from build123d import *

# Parameters (mm, degrees)
SKETCH1_R               = 15
BOSS_EXTRUDE1_DEPTH     = 35
SHELL1_T                = -2
ADVANCEDHOLE1_OUTLINE_R = 3
ADVANCEDHOLE1_DEPTH     = 2


# Read off the part's stored shape, not the designer's step: AdvancedHole1
with BuildPart() as part:
    # Sketch1 → Boss-Extrude1 (new body)
    with BuildSketch(Plane(origin=(0, 0, 0), x_dir=(1, 0, 0), z_dir=(0, 1, 0))):
        with Locations(Location((-13.930579922, 15.357614938, 0), (0, 0, 270))):
            Circle(SKETCH1_R)
    extrude(amount=BOSS_EXTRUDE1_DEPTH)

    # Shell1
    shell1_openings = [part.faces().sort_by_distance(p)[0] for p in [
        (-13.930579922, 35, -15.357614938),
    ]]
    offset(amount=SHELL1_T, openings=shell1_openings, kind=Kind.INTERSECTION)

    # AdvancedHole1 outline → AdvancedHole1 (cut)
    with BuildSketch(Plane(origin=(0, 0, 0), x_dir=(1, 0, 0), z_dir=(0, 1, 0))):
        with Locations((-13.850292644, 15.457974035)):
            Circle(ADVANCEDHOLE1_OUTLINE_R)
    extrude(amount=ADVANCEDHOLE1_DEPTH, mode=Mode.SUBTRACT)


solid = part.part
The model under review builds one solid part; all positions refer to its coordinate system, in mm. A direction names the side the tool comes from. Give positions to 0.01 mm unless a question says otherwise; leave off trailing zeros. Write each loop counter-clockwise with the first axis right and the second up, starting at its lowest first coordinate (ties: lowest second). Pieces come first, ordered by that corner, then holes. Notation, with made-up numbers: M 64.5,3 L 80.5,3 A30 cw 80.5,38 Z; hole C 77,-19.5 d9. An arc over 180 degrees is marked long. One line per question, with ' | ' between items. Start each with the question number.
Item 1: We need section B-B on x = -12.75. Write out the cut boundary in (y, z).
Item 2: We need section C-C on x = -19.75. Write out the cut boundary in (y, z), plus the area to 3 significant figures.
Item 3: Wall thickness on line 1 (X direction, y = 4, z = -15.25); line 2 (Y direction, x = -13.5, z = -6.5); line 3 (X direction, y = 17, z = -6.25): over which ranges is each line inside the solid? List them lowest first. Write a range as from..to.
Item 4: We need section D-D on z = -6.75. Write out the cut boundary in (x, y).
Item 5: For faces 5 (the flat face through (-17, 2, -13)), 6 (the flat face through (-7, 35, -27)), list the 3-axis set-ups (+Z, -Z, +X, -X, +Y, -Y) from which the entire face can be reached by the end or side of a thin tool; tool diameter is ignored.
Item 6: Draft analysis for pull direction X (two halves, no side actions). For faces 1 (the cylindrical face through (-3.79, 17.26, -26.41)), 2 (the cylindrical face through (-16.23, 0.99, -13.63)), 3 (the cylindrical face through (-21.841, 18.269, -25.674)), 4 (the flat face through (-14, 0, -12)), state which applies: released by +X, released by -X, zero draft, split by the parting line, or undercut.
Item 7: We need section A-A on z = -14.5. Write out the cut boundary in (x, y), plus the area to 3 significant figures.
Item 8: For pin 1 (6 mm diameter, centred on x = -20.5, y = 19, fed in from +Z); pin 2 (6 mm diameter, centred on y = 19, z = -4, fed in from +X); pin 3 (3 mm diameter, centred on x = -9.5, y = 5, fed in from -Z), all flat-tipped, find the tip position at first contact; note any pin that passes through.
Results found:
1) outline: M 0,-30.31 L 35,-30.31 L 35,-28.3 L 2,-28.3 L 2,-18.25 L 0,-18.25 Z; M 0,-12.67 L 2,-12.67 L 2,-2.41 L 35,-2.41 L 35,-0.4 L 0,-0.4 Z
2) outline: M 0,-29.18 L 35,-29.18 L 35,-26.98 L 2,-26.98 L 2,-3.73 L 35,-3.73 L 35,-1.53 L 0,-1.53 Z | area: 201 mm2
3) line 1: x = -28.93..-26.93, -0.93..1.07 | line 2: y = 0..2 | line 3: x = -25.85..-23.21, -4.65..-2.01
4) outline: M -26.22,0 L -1.65,0 L -1.65,35 L -4.19,35 L -4.19,2 L -23.67,2 L -23.67,35 L -26.22,35 Z
5) face 5: +Y | face 6: +Z, -Z, +X, -X, +Y
6) face 1: split by the parting line | face 2: undercut | face 3: undercut | face 4: zero draft
7) outline: M -28.91,0 L -16.69,0 L -16.69,2 L -26.9,2 L -26.9,35 L -28.91,35 Z; M -11.01,0 L 1.04,0 L 1.04,35 L -0.96,35 L -0.96,2 L -11.01,2 Z | area: 181 mm2
8) pin 1: stops at z = -0.79 | pin 2: stops at x = -1.47 | pin 3: stops at z = -30.07
